For this review, take the finished solid that the model builds, in its own axes (mm). Face numbers are marked on the shaded views. A direction names the side the tool comes from. Round coordinates to 2 decimals unless told otherwise and drop trailing zeros. Loops run counter-clockwise (first coordinate to the right, second up) from the corner with the lowest first, then second, coordinate; pieces in that order, holes last. Notation, with made-up numbers: (-13.75, 79) -> (-9.75, 79) arc R13 ccw to (-9.75, 86) -> close; hole circle Ø2 at (15, 89.5). An arc over 180 degrees is marked (long way). Write each question's results on one line, items separated by ' | '.
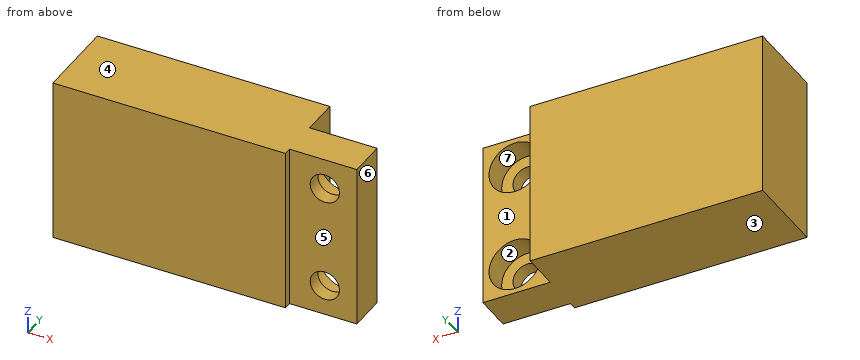
```python
from build123d import *

# Parameters (mm, degrees)
SZKIC1_W                                          = 31.8
SZKIC1_H                                          = 8.8
DODANIE_WYCI_GNI_CIE1_DEPTH                       = 8.75
SZKIC2_W                                          = 7.15
SZKIC2_H                                          = 17.5
WYTNIJ_WYCI_GNI_CIE1_DEPTH                        = 0.8
SZKIC3_W                                          = 7.15
SZKIC3_H                                          = 4
WYTNIJ_WYCI_GNI_CIE2_DEPTH                        = 26.228951623
POG_BIENIE_WALCOWE_POD_M2_5_RUB_Z_BEM_D           = 3.1
POG_BIENIE_WALCOWE_POD_M2_5_RUB_Z_BEM_CBORE_D     = 5.5
POG_BIENIE_WALCOWE_POD_M2_5_RUB_Z_BEM_CBORE_DEPTH = 2.5


with BuildPart() as part:
    # Szkic1 → Dodanie-wyciągnięcie1 (new, symmetric)
    with BuildSketch(Plane.XY):
        with Locations((0, 4.4)):
            Rectangle(SZKIC1_W, SZKIC1_H)
    extrude(amount=DODANIE_WYCI_GNI_CIE1_DEPTH, both=True)

    # Szkic2 → Wytnij-wyciągnięcie1 (cut)
    with BuildSketch(Plane.XZ):
        with Locations((12.325, 0)):
            Rectangle(SZKIC2_W, SZKIC2_H)
    extrude(amount=-WYTNIJ_WYCI_GNI_CIE1_DEPTH, mode=Mode.SUBTRACT)

    # Szkic3 → Wytnij-wyciągnięcie2 (cut, through all)
    with BuildSketch(Plane.XY.offset(8.75)):
        with Locations((12.325, 6.8)):
            Rectangle(SZKIC3_W, SZKIC3_H)
    extrude(amount=-WYTNIJ_WYCI_GNI_CIE2_DEPTH, mode=Mode.SUBTRACT)

    # Pogłębienie walcowe pod M2.5 Śrubę z łbem walcowym z gniazdem1 (through all)
    with Locations(Plane(origin=(0, 4.8, 0), x_dir=(1, 0, 0), z_dir=(0, 1, 0))):
        with Locations((12.5, 5.5), (12.5, -5.5)):
            CounterBoreHole(POG_BIENIE_WALCOWE_POD_M2_5_RUB_Z_BEM_D / 2, POG_BIENIE_WALCOWE_POD_M2_5_RUB_Z_BEM_CBORE_D / 2, POG_BIENIE_WALCOWE_POD_M2_5_RUB_Z_BEM_CBORE_DEPTH)


solid = part.part
```
1. Draft analysis for pull direction Z (two halves, no side actions). For the marked faces 1, 2, 3 and 4, state which applies: released by +Z, released by -Z, zero draft, split by the parting line, or undercut.
Values found:
face 1: zero draft | face 2: undercut | face 3: released by -Z | face 4: released by +Z
2. To check wall thickness, follow probe 1 along Z at (x, y) = (12.5, 4.15); probe 2 along Z at (x, y) = (12.5, 1.9); probe 3 along X at (y, z) = (1.95, 5.5). State the ranges of each line that lie inside material, in increasing order.
Values found:
probe 1: z = -8.75 to -8.25, -2.75 to 2.75, 8.25 to 8.75 | probe 2: z = -8.75 to -7.05, -3.95 to 3.95, 7.05 to 8.75 | probe 3: x = -15.9 to 10.95, 14.05 to 15.9
3. Consider section A-A (x = 12.5). State the section outline as (y, z) points, plus the area to 3 significant figures.
Values found:
outline: (0.8, -8.75) -> (4.8, -8.75) -> (4.8, -8.25) -> (2.3, -8.25) -> (2.3, -7.05) -> (0.8, -7.05) -> close; (0.8, -3.95) -> (2.3, -3.95) -> (2.3, -2.75) -> (4.8, -2.75) -> (4.8, 2.75) -> (2.3, 2.75) -> (2.3, 3.95) -> (0.8, 3.95) -> close; (0.8, 7.05) -> (2.3, 7.05) -> (2.3, 8.25) -> (4.8, 8.25) -> (4.8, 8.75) -> (0.8, 8.75) -> close | area: 33.2 mm2
4. Consider section C-C (y = 4). State the section outline as (x, z) points, plus the area to 3 significant figures.
Values found:
outline: (-15.9, -8.75) -> (15.9, -8.75) -> (15.9, 8.75) -> (-15.9, 8.75) -> close; hole circle Ø5.5 at (12.5, -5.5); hole circle Ø5.5 at (12.5, 5.5) | area: 509 mm2
5. Consider section B-B (z = -5.5). State the section outline as (x, y) points.
Values found:
outline: (-15.9, 0) -> (8.75, 0) -> (8.75, 0.8) -> (10.95, 0.8) -> (10.95, 2.3) -> (9.75, 2.3) -> (9.75, 4.8) -> (8.75, 4.8) -> (8.75, 8.8) -> (-15.9, 8.8) -> close; (14.05, 0.8) -> (15.9, 0.8) -> (15.9, 4.8) -> (15.25, 4.8) -> (15.25, 2.3) -> (14.05, 2.3) -> close
6. Tool access review of the marked faces 5, 6 and 7: name each direction out of +Z, -Z, +X, -X, +Y, -Y from which nothing blocks a thin tool from reaching the whole face with its end or side.
Values found:
face 5: +Z, -Z, +X, -Y | face 6: +Z, -Z, +X, +Y, -Y | face 7: +Y
7. For pin 1 (7 mm diameter, centred on x = 12.5, z = 5.5, fed in from +Y); pin 2 (1.2 mm diameter, centred on y = 6, z = 0, fed in from +X); pin 3 (3 mm diameter, centred on x = 13, z = 6.5, fed in from +Y), all flat-tipped, find the tip position at first contact; note any pin that passes through.
Values found:
pin 1: stops at y = 4.8 | pin 2: stops at x = 8.75 | pin 3: stops at y = 2.3
8. Consider section D-D (y = 5.5). State the section outline as (x, z) points, plus the area to 3 significant figures.
Values found:
outline: (-15.9, -8.75) -> (8.75, -8.75) -> (8.75, 8.75) -> (-15.9, 8.75) -> close | area: 431 mm2
